CAD build for the part. Positions are in the model's coordinates, mm. Coordinates: 2 decimals unless noted, no trailing zeros. Loops run counter-clockwise (first coordinate to the right, second up) from the corner with the lowest first, then second, coordinate; pieces in that order, holes last. Notation, with made-up numbers: (88, -3.75) -> (109, -3.75) arc R16 cw to (109, 15.25) -> close; hole circle Ø2 at (-25, -27.75). An arc over 180 degrees is marked (long way). Answer as CSV lines item,"result". Start each with the question number.
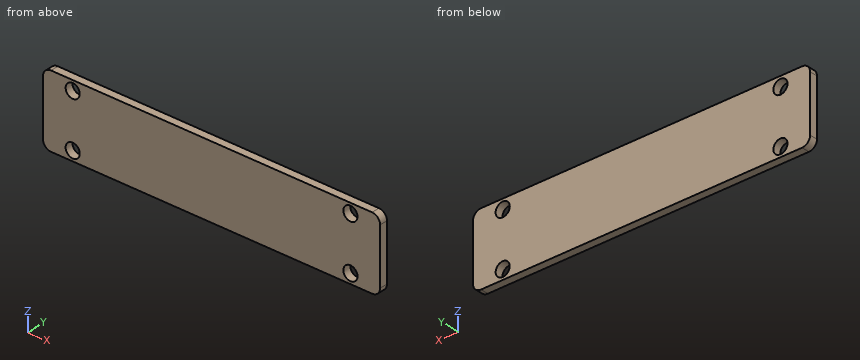
```python
from build123d import *

# Parameters (mm, degrees)
F0_W     = 210
F0_H     = 45
F1_DEPTH = 5
F3_D     = 8.8
F4_R     = 5


with BuildPart() as f1:
    # F0 (on Front) → F1 (new body)
    with BuildSketch(Plane.XZ):
        with Locations((105, 22.5)):
            Rectangle(F0_W, F0_H)
    extrude(amount=F1_DEPTH)

    # F3 (through all)
    with Locations(Plane.XZ.offset(5)):
        with Locations((18.5, 39), (18.5, 6), (191.5, 39), (191.5, 6)):
            Hole(F3_D / 2)

    # F4
    f4_edges = [f1.edges().sort_by_distance(p)[0] for p in [
        (0, -2.5, 45),
        (0, -2.5, 0),
        (210, -2.5, 0),
        (210, -2.5, 45),
    ]]
    fillet(f4_edges, radius=F4_R)


solid = f1.part
```
Q1. Pin check, flat tip, straight feed: pin 1 Ø7 at (x, z) = (191.5, 6) entering from +Y. Stop position of the tip, or through.
Q2. Saw through at B-B (x = 18.5). List the corners of the cut face in (y, z), and give its area (3 significant figures).
Q3. Saw through at A-A (y = -1.6). List the corners of the cut face in (x, z).
Q4. Probe probe 1 along Z at (x, y) = (18.5, -2.8); probe 2 along X at (y, z) = (-2.2, 38); probe 3 along Z at (x, y) = (17, -2.05). List the from-to ranges inside material, lowest first. Write a range as from..to.
Ans:
1,pin 1,"passes through"
2,outline,"(-5, 0) -> (0, 0) -> (0, 1.6) -> (-5, 1.6) -> close; (-5, 10.4) -> (0, 10.4) -> (0, 34.6) -> (-5, 34.6) -> close; (-5, 43.4) -> (0, 43.4) -> (0, 45) -> (-5, 45) -> close"
2,area,"137 mm²"
3,outline,"(0, 5) arc R5 ccw to (5, 0) -> (205, 0) arc R5 ccw to (210, 5) -> (210, 40) arc R5 ccw to (205, 45) -> (5, 45) arc R5 ccw to (0, 40) -> close; hole circle Ø8.8 at (18.5, 6); hole circle Ø8.8 at (18.5, 39); hole circle Ø8.8 at (191.5, 6); hole circle Ø8.8 at (191.5, 39)"
4,probe 1,"z = 0..1.6, 10.4..34.6, 43.4..45"
4,probe 2,"x = 0..14.22, 22.78..187.22, 195.78..210"
4,probe 3,"z = 0..1.86, 10.14..34.86, 43.14..45"
